Could you check a few things on this model? Use its own coordinates, in mm. A direction names the side the tool comes from. Round coordinates to 2 decimals unless told otherwise and drop trailing zeros. Write each loop counter-clockwise with the first axis right and the second up, starting at its lowest first coordinate (ties: lowest second). Pieces come first, ordered by that corner, then holes. Notation, with made-up numbers: (-6, -36.5) - (48, -36.5) arc R14 ccw to (48, -22.5) - close; hole circle Ø8 at (37, 72). An arc over 180 degrees is marked (long way). Put each result on its own line as item: value.
from build123d import *

# Parameters (mm, degrees)
SKETCH1_W               = 75
SKETCH1_H               = 100
BOSS_EXTRUDE1_DEPTH     = 2
CUT_EXTRUDE1_REACH      = 4
SKETCH2_W               = 10
SKETCH2_H               = 50
SKETCH3_W               = 1.75
SKETCH3_H               = 10
BOSS_EXTRUDE2_DEPTH     = 2
BOSS_EXTRUDE3_DEPTH     = 15
SKETCH5_R               = 1.75
CUT_EXTRUDE2_DEPTH      = 65
CUT_EXTRUDE2_DEPTH_BACK = 12


with BuildPart() as part:
    # Sketch1 → Boss-Extrude1 (new body)
    with BuildSketch(Plane(origin=(0, 0, 0), x_dir=(1, 0, 0), z_dir=(0, 1, 0))):
        Rectangle(SKETCH1_W, SKETCH1_H)
    extrude(amount=BOSS_EXTRUDE1_DEPTH)

    # Sketch2 → Cut-Extrude1 (cut, up to next)
    with BuildSketch(Plane(origin=(0, 2, 0), x_dir=(1, 0, 0), z_dir=(0, 1, 0)), mode=Mode.PRIVATE) as cut_extrude1_sk1:
        with Locations((26.5, 0)):
            Rectangle(SKETCH2_W, SKETCH2_H)
    cut_extrude1_tool1 = extrude(cut_extrude1_sk1.sketch, amount=-CUT_EXTRUDE1_REACH, mode=Mode.PRIVATE) & part.part
    add(cut_extrude1_tool1.solids().sort_by_distance((26.5, 2, 0))[0], mode=Mode.SUBTRACT)

    # Sketch3 → Boss-Extrude2 (add)
    with BuildSketch(Plane.XZ):
        with Locations((22.375, 20)):
            Rectangle(SKETCH3_W, SKETCH3_H)
        with Locations((30.625, 20)):
            Rectangle(SKETCH3_W, SKETCH3_H)
    extrude(amount=-BOSS_EXTRUDE2_DEPTH)

    # Sketch4 → Boss-Extrude3 (add)
    with BuildSketch(Plane.XZ):
        Polygon((33.5, 17), (31.75, 17), (31.75, 27), (21.25, 27), (21.25, 17), (19.5, 17), (19.5, -27), (33.5, -27), align=None)
        Polygon((31.5, 15), (29.75, 15), (29.75, 25), (23.25, 25), (23.25, 15), (21.5, 15), (21.5, -25), (31.5, -25), align=None, mode=Mode.SUBTRACT)
    extrude(amount=BOSS_EXTRUDE3_DEPTH)

    # Sketch5 → Cut-Extrude2 (cut, two sides)
    with BuildSketch(Plane.ZY.offset(-26.5)) as cut_extrude2_sk:
        with Locations((22, -3.5)):
            Circle(SKETCH5_R)
    extrude(amount=CUT_EXTRUDE2_DEPTH, mode=Mode.SUBTRACT)
    extrude(cut_extrude2_sk.sketch, amount=-CUT_EXTRUDE2_DEPTH_BACK, mode=Mode.SUBTRACT)


solid = part.part
(1) For faces 1 (the face through (26, -7, -27)), 2 (the face through (19.5, -7, -5)), 3 (the face through (33.5, -7, -5)), 4 (the face through (29.75, -6, 20)), which set-ups out of +Z, -Z, +X, -X, +Y, -Y let a thin tool reach every point of the face, with its end or its side?
Values found:
face 1: -Z, +X, -X, -Y
face 2: +Z, -Z, -X, -Y
face 3: +Z, -Z, +X, -Y
face 4: +Y, -Y
(2) Imagine slicing it at A-A, the plane z = 3.5. List the corners of the cut face in (x, y) for me.
Values found:
outline: (-37.5, 0) - (19.5, 0) - (19.5, -15) - (21.5, -15) - (21.5, 2) - (-37.5, 2) - close; (31.5, -15) - (33.5, -15) - (33.5, 0) - (37.5, 0) - (37.5, 2) - (31.5, 2) - close
(3) Imagine slicing it at C-C, the plane y = -3.5. List the corners of the cut face in (x, z) for me.
Values found:
outline: (19.5, -27) - (33.5, -27) - (33.5, 17) - (31.75, 17) - (31.75, 20.25) - (29.75, 20.25) - (29.75, 15) - (31.5, 15) - (31.5, -25) - (21.5, -25) - (21.5, 15) - (23.25, 15) - (23.25, 20.25) - (21.25, 20.25) - (21.25, 17) - (19.5, 17) - close; (21.25, 23.75) - (23.25, 23.75) - (23.25, 25) - (29.75, 25) - (29.75, 23.75) - (31.75, 23.75) - (31.75, 27) - (21.25, 27) - close
(4) Please list where these lines run through material, in increasing order: probe 1 along X at (y, z) = (-0.5, 23.5); probe 2 along Z at (x, y) = (29.5, -12.75); probe 3 along X at (y, z) = (0.5, -10.5). Write a range as from..to.
Values found:
probe 1: x = 21.25..23.25, 29.75..31.75
probe 2: z = -27..-25, 25..27
probe 3: x = -37.5..21.5, 31.5..37.5
(5) Imagine slicing it at B-B, the plane y = -8.5. List the corners of the cut face in (x, z) for me.
Values found:
outline: (19.5, -27) - (33.5, -27) - (33.5, 17) - (31.75, 17) - (31.75, 27) - (21.25, 27) - (21.25, 17) - (19.5, 17) - close; hole (21.5, -25) - (31.5, -25) - (31.5, 15) - (29.75, 15) - (29.75, 25) - (23.25, 25) - (23.25, 15) - (21.5, 15) - close
(6) I'm going to push flat-ended pins straight in: pin 1 (3 mm diameter, centred on y = -5.5, z = 24, fed in from -X); pin 2 (1.4 mm diameter, centred on x = 30.5, y = -7.5, fed in from -Z); pin 3 (1.5 mm diameter, centred on y = -7.5, z = 6, fed in from -X). Where does each tip first touch, or does it pass through?
Values found:
pin 1: stops at x = 21.25
pin 2: stops at z = -27
pin 3: stops at x = 19.5
(7) Imagine slicing it at D-D, the plane z = 22. List the corners of the cut face in (x, y) for me.
Values found:
outline: (-37.5, 0) - (21.25, 0) - (21.25, -1.75) - (23.25, -1.75) - (23.25, 2) - (-37.5, 2) - close; (21.25, -15) - (23.25, -15) - (23.25, -5.25) - (21.25, -5.25) - close; (29.75, -15) - (31.75, -15) - (31.75, -5.25) - (29.75, -5.25) - close; (29.75, -1.75) - (31.75, -1.75) - (31.75, 0) - (37.5, 0) - (37.5, 2) - (29.75, 2) - close
(8) If we mould it in two halves opening along X, with no side actions, what happens to faces 5 (the face through (-1, 1, -50)), 6 (the face through (27, -6, 25)), 7 (the face through (-37.5, 1, 1)), 8 (the face through (31.5, -6, -5))? For each: pulls with the +X half, pulls with the -X half, needs draft (parallel to the pull), parting line crosses it, or undercut.
Values found:
face 5: needs draft
face 6: undercut
face 7: pulls with the -X half
face 8: undercut
